The listing builds one solid part. Answer for the finished solid, in the listing's coordinates (mm). A direction names the side the tool comes from. Round coordinates to 2 decimals unless told otherwise and drop trailing zeros. Write each loop counter-clockwise with the first axis right and the second up, starting at its lowest first coordinate (ties: lowest second). Pieces come first, ordered by that corner, then holes. Notation, with made-up numbers: (80, 2.25) - (103, 2.25) arc R17 cw to (103, 9.25) - close; hole circle Ø7 at (26, 13). An arc over 180 degrees is marked (long way). Answer in a Markdown table with one row per item.
from build123d import *

# Parameters (mm, degrees)
F0_R     = 15
F1_DEPTH = 30
F2_DEPTH = 5


with BuildPart() as f1:
    # F0 (on Top) → F1 (new body)
    with BuildSketch(Plane.XY):
        Circle(F0_R)
        with BuildLine():
            Line((-6.866588, 4.182289), (6.866588, 4.182289))
            ThreePointArc((6.866588, 4.182289), (11.048877, 0), (6.866588, -4.182289))
            Line((6.866588, -4.182289), (-6.866588, -4.182289))
            ThreePointArc((-6.866588, -4.182289), (-11.048877, 0), (-6.866588, 4.182289))
        make_face(mode=Mode.SUBTRACT)
    extrude(amount=F1_DEPTH)

    # F0 (on Top) → F2 (join)
    with BuildSketch(Plane.XY):
        with BuildLine():
            ThreePointArc((6.866588, -4.182289), (11.048877, 0), (6.866588, 4.182289))
            Line((6.866588, 4.182289), (-6.866588, 4.182289))
            ThreePointArc((-6.866588, 4.182289), (-11.048877, 0), (-6.866588, -4.182289))
            Line((-6.866588, -4.182289), (6.866588, -4.182289))
        make_face()
        with BuildLine():
            ThreePointArc((6.866588, -0.319086), (6.547502, 0), (6.866588, 0.319086))
            ThreePointArc((6.866588, 0.319086), (7.092216, 0.225628), (7.185674, 0))
            ThreePointArc((7.185674, 0), (7.092216, -0.225628), (6.866588, -0.319086))
        make_face(mode=Mode.SUBTRACT)
    extrude(amount=F2_DEPTH)


solid = f1.part
(1) Find the intervals of material crossed by line 1 (Y direction, x = -0.5, z = 13.5); line 2 (Y direction, x = -0.5, z = 4.5); line 3 (Z direction, x = 5.75, y = 4), in increasing order.
Checked values:
| item | result |
|---|---|
| line 1 | y = -14.99 to -4.18, 4.18 to 14.99 |
| line 2 | y = -14.99 to 14.99 |
| line 3 | z = 0 to 5 |
(2) Section D-D (y = -12) is taken. Give the vertices of the cut face in (x, z).
Checked values:
| item | result |
|---|---|
| outline | (-9, 0) - (9, 0) - (9, 30) - (-9, 30) - close |
(3) Flat-ended cylindrical pins translate along their axes: pin 1 (4 mm diameter, centred on x = -3, z = 23, fed in from -Y); pin 2 (10 mm diameter, centred on x = 7.5, z = 15, fed in from +Y); pin 3 (3 mm diameter, centred on x = 6.5, z = 18, fed in from -Y). Find the tip coordinate at first contact, or state that the pin passes through.
Checked values:
| item | result |
|---|---|
| pin 1 | stops at y = -14.97 |
| pin 2 | stops at y = 14.79 |
| pin 3 | stops at y = -14.14 |
(4) Section A-A (z = 6.25) is taken. Give the vertices of the cut face in (x, y).
Checked values:
| item | result |
|---|---|
| outline | circle Ø30 at (0, 0); hole (-6.87, -4.18) - (6.87, -4.18) arc R4.18 ccw to (6.87, 4.18) - (-6.87, 4.18) arc R4.18 ccw to start |
(5) For a pull along X with two mould halves and no side action, classify faces 1 (the cylindrical face through (-11.048, -0.092, 17.325)), 2 (the flat face through (0, 0, 0)), 3 (the flat face through (0, -4.182, 17)), 4 (the cylindrical face through (-14.985, 0.66, 14.79)) as pulls with the +X half, pulls with the -X half, needs draft (parallel to the pull), parting line crosses it, or undercut.
Checked values:
| item | result |
|---|---|
| face 1 | undercut |
| face 2 | needs draft |
| face 3 | undercut |
| face 4 | parting line crosses it |
(6) Section B-B (x = 0) is taken. Give the vertices of the cut face in (y, z).
Checked values:
| item | result |
|---|---|
| outline | (-15, 0) - (15, 0) - (15, 30) - (4.18, 30) - (4.18, 5) - (-4.18, 5) - (-4.18, 30) - (-15, 30) - close |
(7) Section C-C (y = -3.5) is taken. Give the vertices of the cut face in (x, z).
Checked values:
| item | result |
|---|---|
| outline | (-14.59, 0) - (14.59, 0) - (14.59, 30) - (9.16, 30) - (9.16, 5) - (-9.16, 5) - (-9.16, 30) - (-14.59, 30) - close |
(8) For faces 5 (the flat face through (0, -6, 30)), 6 (the flat face through (0, 0, 5)), determine the directions among +Z, -Z, +X, -X, +Y, -Y from which every point of the face is accessible in a straight line to the end or side of a thin tool.
Checked values:
| item | result |
|---|---|
| face 5 | +Z, +X, -X, +Y, -Y |
| face 6 | +Z |
